Build history of the part. All positions in model axes, mm. Round coordinates to 2 decimals unless told otherwise and drop trailing zeros. Write each loop counter-clockwise with the first axis right and the second up, starting at its lowest first coordinate (ties: lowest second). Pieces come first, ordered by that corner, then holes. Notation, with made-up numbers: (59, 77) - (63, 77) arc R18 cw to (63, 81) - close; hole circle Ø3 at (-33, -27.75). An arc over 180 degrees is marked (long way). One line per question, with ' | ' between items.
Autodesk Inventor part; units mm, degrees
ref_plane "YZ Plane" through (0, 0, 0) normal (1, 0, 0) x (0, 1, 0)
ref_plane "XZ Plane" through (0, 0, 0) normal (0, 1, 0) x (-1, 0, 0)
ref_plane "XY Plane" through (0, 0, 0) normal (0, 0, 1) x (1, 0, 0)
sketch "Sketch1" plane through (0, 0, 0) normal (1, 0, 0) x (0, 1, 0)
  line L0 (80, -25) -> (-80, -25)
  line L1 (-80, -25) -> (-80, 25)
  line L2 (-80, 25) -> (80, 25)
  line L3 (80, 25) -> (80, -25)
  line L4 (80, -25) -> (-80, 25) construction
  line L5 (-80, -25) -> (80, 25) construction
  point P0 (0, 0)
  dimension "d0" = 160
  dimension "d1" = 50
extrude "Extrusion1" add sketch "Sketch1" along normal blind 6
sketch "Sketch2" plane through (6, 0, 0) normal (1, 0, 0) x (0, 0, -1)
  line L0 (-25, 80) -> (-25, -80)
  line L1 (-25, 80) -> (-31, 80)
  line L2 (-31, 80) -> (-31, 43.5)
  line L3 (-31, 43.5) -> (-25, 43.5)
  line L4 (-25, 43.5) -> (-25, 80)
  line L5 (-25, 18.25) -> (-31, 18.25)
  line L6 (-31, 18.25) -> (-31, -18.25)
  line L7 (-31, -18.25) -> (-25, -18.25)
  line L8 (-25, -18.25) -> (-25, 18.25)
  line L9 (-25, -80) -> (-31, -80)
  line L10 (-31, -80) -> (-31, -43.5)
  line L11 (-31, -43.5) -> (-25, -43.5)
  line L12 (-25, -43.5) -> (-25, -80)
  point P0 (0, 0)
  dimension "d4" = 6
  dimension "d5" = 25.25
  dimension "d6" = 25.25
extrude "Extrusion2" add sketch "Sketch2" against normal blind 6
sketch "Sketch3" plane through (6, 0, 0) normal (1, 0, 0) x (0, 0, -1)
  line L0 (-25, 43.5) -> (-25, 18.25)
  line L1 (-31, -80) -> (25, -80)
  line L2 (-25, 30.875) -> (0, 30.875) construction
  line L3 (-25, 29.825) -> (-25, 31.925)
  line L4 (-25, 31.925) -> (-19, 31.925)
  line L5 (-19, 31.925) -> (-19, 32.925)
  line L6 (-19, 32.925) -> (-17.2, 32.925)
  line L7 (-17.2, 32.925) -> (-17.2, 31.925)
  line L8 (-17.2, 31.925) -> (-16, 31.925)
  line L9 (-16, 31.925) -> (-16, 29.825)
  line L10 (-16, 29.825) -> (-17.2, 29.825)
  line L11 (-17.2, 29.825) -> (-17.2, 28.825)
  line L12 (-17.2, 28.825) -> (-19, 28.825)
  line L13 (-19, 28.825) -> (-19, 29.825)
  line L14 (-19, 29.825) -> (-25, 29.825)
  point P0 (0, 0)
  dimension "d9" = 1.8
  dimension "d10" = 4.1
  dimension "d11" = 2.1
  dimension "d12" = 1.05
  dimension "d13" = 9
  dimension "d14" = 2.05
  dimension "d15" = 6
extrude "Extrusion3" cut sketch "Sketch3" against normal through all
mirror "Mirror1" about plane through (0, 0, 0) normal (0, 1, 0) of "Extrusion3"
fillet "Fillet1" radius 2 8 edges at (3, 43.5, 31) (3, 80, 31) (3, 18.25, 31) (3, -18.25, 31) (3, -43.5, 31) (3, -80, 31) (3, 80, -25) (3, -80, -25)
equation "\"d12\" = 0.5 * d11"
equation "\"d14\" = 0.5 * d10"
properties part number "InnerSide"
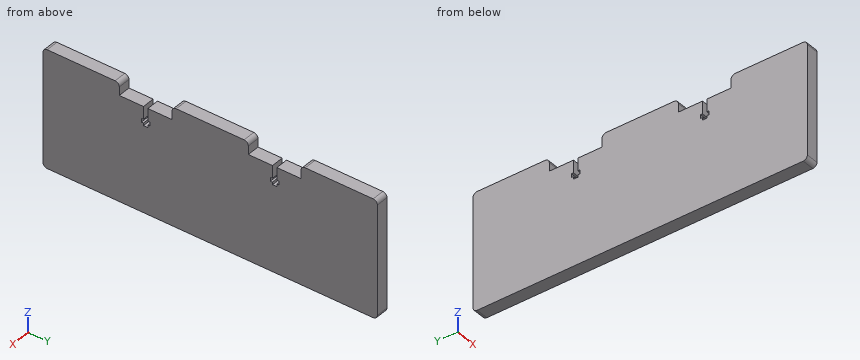
Q1. Drop flat-ended pins along their axis: pin 1 (0.5 mm diameter, centred on x = 3, y = 32.5, fed in from +Z); pin 2 (2 mm diameter, centred on y = 29, z = -0.5, fed in from -X); pin 3 (1.7 mm diameter, centred on x = 4, y = -31, fed in from +Z). Give the stop position or say it passes through.
Found:
pin 1: z = 25 | pin 2: x = 0 | pin 3: z = 16
Q2. Saw through at A-A, the plane y = -41. List the corners of the cut face in (x, z), then the cut area to 3 significant figures.
Found:
outline: (0, -25) - (6, -25) - (6, 25) - (0, 25) - close | area: 300 mm^2
Q3. Drill centre lines: L1, parallel to Y at x = 1.55, z = 18.5 (3 decimals); L2, parallel to Y at x = 1.1, z = 26; L3, parallel to Z at x = 3.3, y = 39. Where is each one in solid material? Low to high. Write a range as from..to.
Found:
L1: -80..-32.925, -28.825..28.825, 32.925..80 | L2: -80..-43.5, -18.25..18.25, 43.5..80 | L3: -25..25
